Read the model definition and answer for the solid it produces. Units are mm, in the model's axes. Face numbers are marked on the shaded views. A direction names the side the tool comes from. Give positions to 0.01 mm unless a question says otherwise; leave off trailing zeros. Order: outer loops, then holes, each group sorted by start corner. A loop starts at its lowest first (then second) coordinate and runs counter-clockwise, first axis right, second up. Notation, with made-up numbers: (-10, 36) - (43, 36) arc R25 cw to (43, 51) - close; hole circle Ø2 at (5, -16). An arc over 180 degrees is marked (long way). Return JSON: item names as keys, results as strings.
```python
from build123d import *

# Parameters (mm, degrees)
SKETCH1_W                    = 410
SKETCH1_H                    = 200
BASE_FLANGE1_DEPTH           = 2
EDGE_FLANGE2_STRIP_W         = 13
EDGE_FLANGE2_STRIP_H         = 2
EDGE_FLANGE2_STRIP_CUT_DEPTH = 200
EDGE_FLANGE2_DEPTH           = 200
EDGE_FLANGE4_STRIP_W         = 13
EDGE_FLANGE4_STRIP_H         = 2
EDGE_FLANGE4_STRIP_CUT_DEPTH = 200
EDGE_FLANGE4_DEPTH           = 200
EDGE_FLANGE5_STRIP_W         = 13
EDGE_FLANGE5_STRIP_H         = 2
EDGE_FLANGE5_STRIP_CUT_DEPTH = 200
EDGE_FLANGE5_DEPTH           = 200
EDGE_FLANGE6_STRIP_W         = 13
EDGE_FLANGE6_STRIP_H         = 2
EDGE_FLANGE6_STRIP_CUT_DEPTH = 403
EDGE_FLANGE6_DEPTH           = 403
EDGE_FLANGE7_STRIP_W         = 13
EDGE_FLANGE7_STRIP_H         = 2
EDGE_FLANGE7_STRIP_CUT_DEPTH = 403
EDGE_FLANGE7_DEPTH           = 403
EDGE_FLANGE8_STRIP_W         = 13
EDGE_FLANGE8_STRIP_H         = 2
EDGE_FLANGE8_STRIP_CUT_DEPTH = 407.5
EDGE_FLANGE8_DEPTH           = 407.5
EDGE_FLANGE9_STRIP_W         = 13
EDGE_FLANGE9_STRIP_H         = 2
EDGE_FLANGE9_STRIP_CUT_DEPTH = 404.5
EDGE_FLANGE9_DEPTH           = 404.5
SKETCH29_R                   = 52.5
CUT_EXTRUDE1_DEPTH           = 10
SKETCH30_R                   = 3.25
CUT_EXTRUDE2_DEPTH           = 10


# Sheet-metal steps are written as plain solids
with BuildPart() as part:
    # Sketch1 → Base-Flange1 (new body)
    with BuildSketch(Plane.XY):
        with Locations((-14.494949495, 3.017676768)):
            Rectangle(SKETCH1_W, SKETCH1_H)
    extrude(amount=-BASE_FLANGE1_DEPTH)

    # Edge-Flange2 strip (across the edge) → Edge-Flange2 strip cut (cut)
    with BuildSketch(Plane(origin=(190.505050505, 103.017676768, -2), x_dir=(-1, 0, 0), z_dir=(0, -1, 0))):
        with Locations((-4, -1)):
            Rectangle(EDGE_FLANGE2_STRIP_W, EDGE_FLANGE2_STRIP_H)
    extrude(amount=EDGE_FLANGE2_STRIP_CUT_DEPTH, mode=Mode.SUBTRACT)

    # Edge-Flange2 section (across the edge) → Edge-Flange2 (add)
    with BuildSketch(Plane(origin=(190.505050505, 103.017676768, -2), x_dir=(-1, 0, 0), z_dir=(0, -1, 0))):
        with BuildLine():
            Line((-2, 2.5), (-2, 408))
            Line((-2, 408), (0, 408))
            Line((0, 408), (0, 2.5))
            ThreePointArc((0, 2.5), (0.732233047, 0.732233047), (2.5, 0))
            Line((2.5, 0), (2.5, -2))
            ThreePointArc((2.5, -2), (-0.681980515, -0.681980515), (-2, 2.5))
        make_face()
    extrude(amount=EDGE_FLANGE2_DEPTH)

    # Edge-Flange4 strip (across the edge) → Edge-Flange4 strip cut (cut)
    with BuildSketch(Plane(origin=(190.505050505, 103.017676768, -410), x_dir=(0, 0, 1), z_dir=(0, -1, 0))):
        with Locations((-4, -1)):
            Rectangle(EDGE_FLANGE4_STRIP_W, EDGE_FLANGE4_STRIP_H)
    extrude(amount=EDGE_FLANGE4_STRIP_CUT_DEPTH, mode=Mode.SUBTRACT)

    # Edge-Flange4 section (across the edge) → Edge-Flange4 (add)
    with BuildSketch(Plane(origin=(190.505050505, 103.017676768, -410), x_dir=(0, 0, 1), z_dir=(0, -1, 0))):
        with BuildLine():
            Line((-2, 2.5), (-2, 408))
            Line((-2, 408), (0, 408))
            Line((0, 408), (0, 2.5))
            ThreePointArc((0, 2.5), (0.732233047, 0.732233047), (2.5, 0))
            Line((2.5, 0), (2.5, -2))
            ThreePointArc((2.5, -2), (-0.681980515, -0.681980515), (-2, 2.5))
        make_face()
    extrude(amount=EDGE_FLANGE4_DEPTH)

    # Edge-Flange5 strip (across the edge) → Edge-Flange5 strip cut (cut)
    with BuildSketch(Plane(origin=(-217.494949495, 103.017676768, -410), x_dir=(1, 0, 0), z_dir=(0, -1, 0))):
        with Locations((-4, -1)):
            Rectangle(EDGE_FLANGE5_STRIP_W, EDGE_FLANGE5_STRIP_H)
    extrude(amount=EDGE_FLANGE5_STRIP_CUT_DEPTH, mode=Mode.SUBTRACT)

    # Edge-Flange5 section (across the edge) → Edge-Flange5 (add)
    with BuildSketch(Plane(origin=(-217.494949495, 103.017676768, -410), x_dir=(1, 0, 0), z_dir=(0, -1, 0))):
        with BuildLine():
            Line((-2, 2.5), (-2, 407))
            Line((-2, 407), (0, 407))
            Line((0, 407), (0, 2.5))
            ThreePointArc((0, 2.5), (0.732233047, 0.732233047), (2.5, 0))
            Line((2.5, 0), (2.5, -2))
            ThreePointArc((2.5, -2), (-0.681980515, -0.681980515), (-2, 2.5))
        make_face()
    extrude(amount=EDGE_FLANGE5_DEPTH)

    # Edge-Flange6 strip (across the edge) → Edge-Flange6 strip cut (cut)
    with BuildSketch(Plane(origin=(188.005050505, -96.982323232, -412), x_dir=(0, 1, 0), z_dir=(-1, 0, 0))):
        with Locations((-4, -1)):
            Rectangle(EDGE_FLANGE6_STRIP_W, EDGE_FLANGE6_STRIP_H)
    extrude(amount=EDGE_FLANGE6_STRIP_CUT_DEPTH, mode=Mode.SUBTRACT)

    # Edge-Flange6 section (across the edge) → Edge-Flange6 (add)
    with BuildSketch(Plane(origin=(188.005050505, -96.982323232, -412), x_dir=(0, 1, 0), z_dir=(-1, 0, 0))):
        with BuildLine():
            Line((-2, 2.5), (-2, 18))
            Line((-2, 18), (0, 18))
            Line((0, 18), (0, 2.5))
            ThreePointArc((0, 2.5), (0.732233047, 0.732233047), (2.5, 0))
            Line((2.5, 0), (2.5, -2))
            ThreePointArc((2.5, -2), (-0.681980515, -0.681980515), (-2, 2.5))
        make_face()
    extrude(amount=EDGE_FLANGE6_DEPTH)

    # Edge-Flange7 strip (across the edge) → Edge-Flange7 strip cut (cut)
    with BuildSketch(Plane(origin=(192.505050505, -96.982323232, -4.5), x_dir=(0, 1, 0), z_dir=(0, 0, -1))):
        with Locations((-4, -1)):
            Rectangle(EDGE_FLANGE7_STRIP_W, EDGE_FLANGE7_STRIP_H)
    extrude(amount=EDGE_FLANGE7_STRIP_CUT_DEPTH, mode=Mode.SUBTRACT)

    # Edge-Flange7 section (across the edge) → Edge-Flange7 (add)
    with BuildSketch(Plane(origin=(192.505050505, -96.982323232, -4.5), x_dir=(0, 1, 0), z_dir=(0, 0, -1))):
        with BuildLine():
            Line((-2, 2.5), (-2, 18))
            Line((-2, 18), (0, 18))
            Line((0, 18), (0, 2.5))
            ThreePointArc((0, 2.5), (0.732233047, 0.732233047), (2.5, 0))
            Line((2.5, 0), (2.5, -2))
            ThreePointArc((2.5, -2), (-0.681980515, -0.681980515), (-2, 2.5))
        make_face()
    extrude(amount=EDGE_FLANGE7_DEPTH)

    # Edge-Flange8 strip (across the edge) → Edge-Flange8 strip cut (cut)
    with BuildSketch(Plane(origin=(-219.494949495, -96.982323232, 0), x_dir=(0, 1, 0), z_dir=(1, 0, 0))):
        with Locations((-4, -1)):
            Rectangle(EDGE_FLANGE8_STRIP_W, EDGE_FLANGE8_STRIP_H)
    extrude(amount=EDGE_FLANGE8_STRIP_CUT_DEPTH, mode=Mode.SUBTRACT)

    # Edge-Flange8 section (across the edge) → Edge-Flange8 (add)
    with BuildSketch(Plane(origin=(-219.494949495, -96.982323232, 0), x_dir=(0, 1, 0), z_dir=(1, 0, 0))):
        with BuildLine():
            Line((-2, 2.5), (-2, 18))
            Line((-2, 18), (0, 18))
            Line((0, 18), (0, 2.5))
            ThreePointArc((0, 2.5), (0.732233047, 0.732233047), (2.5, 0))
            Line((2.5, 0), (2.5, -2))
            ThreePointArc((2.5, -2), (-0.681980515, -0.681980515), (-2, 2.5))
        make_face()
    extrude(amount=EDGE_FLANGE8_DEPTH)

    # Edge-Flange9 strip (across the edge) → Edge-Flange9 strip cut (cut)
    with BuildSketch(Plane(origin=(-219.494949495, -96.982323232, -407.5), x_dir=(0, 1, 0), z_dir=(0, 0, 1))):
        with Locations((-4, -1)):
            Rectangle(EDGE_FLANGE9_STRIP_W, EDGE_FLANGE9_STRIP_H)
    extrude(amount=EDGE_FLANGE9_STRIP_CUT_DEPTH, mode=Mode.SUBTRACT)

    # Edge-Flange9 section (across the edge) → Edge-Flange9 (add)
    with BuildSketch(Plane(origin=(-219.494949495, -96.982323232, -407.5), x_dir=(0, 1, 0), z_dir=(0, 0, 1))):
        with BuildLine():
            Line((-2, 2.5), (-2, 18))
            Line((-2, 18), (0, 18))
            Line((0, 18), (0, 2.5))
            ThreePointArc((0, 2.5), (0.732233047, 0.732233047), (2.5, 0))
            Line((2.5, 0), (2.5, -2))
            ThreePointArc((2.5, -2), (-0.681980515, -0.681980515), (-2, 2.5))
        make_face()
    extrude(amount=EDGE_FLANGE9_DEPTH)

    # Sketch29 → Cut-Extrude1 (cut)
    with BuildSketch(Plane.XY):
        with Locations((-15.744949495, 4.267676768)):
            Circle(SKETCH29_R)
    extrude(amount=-CUT_EXTRUDE1_DEPTH, mode=Mode.SUBTRACT)

    # Sketch30 → Cut-Extrude2 (cut)
    with BuildSketch(Plane(origin=(0, -96.982323232, 0), x_dir=(1, 0, 0), z_dir=(0, 1, 0))):
        with Locations(Location((-83.994949495, -10.25, 0), (0, 0, 270))):
            Circle(SKETCH30_R)
        with Locations(Location((52.505050505, -10.25, 0), (0, 0, 270))):
            Circle(SKETCH30_R)
        with Locations(Location((202.755050505, 140, 0), (0, 0, 270))):
            Circle(SKETCH30_R)
        with Locations(Location((202.755050505, 276.5, 0), (0, 0, 270))):
            Circle(SKETCH30_R)
        with Locations(Location((52.505050505, 422.25, 0), (0, 0, 270))):
            Circle(SKETCH30_R)
        with Locations(Location((-83.994949495, 422.25, 0), (0, 0, 270))):
            Circle(SKETCH30_R)
        with Locations(Location((-229.744949495, 272, 0), (0, 0, 270))):
            Circle(SKETCH30_R)
        with Locations(Location((-229.744949495, 135.5, 0), (0, 0, 270))):
            Circle(SKETCH30_R)
    extrude(amount=-CUT_EXTRUDE2_DEPTH, mode=Mode.SUBTRACT)


solid = part.part
```
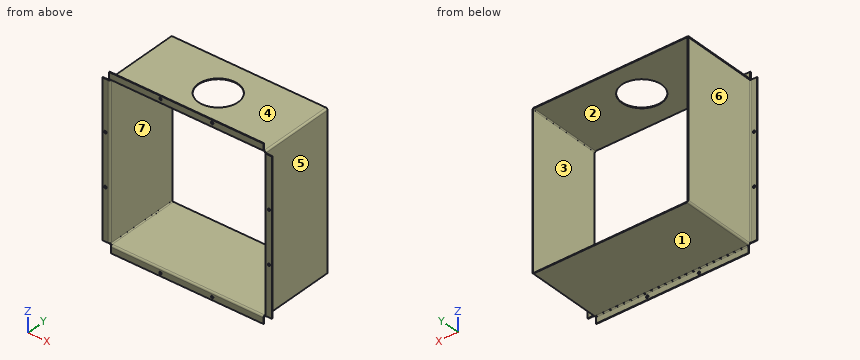
Q1. Given pin 1 (3.5 mm diameter, centred on x = 191.5, z = -409, fed in from -Y); pin 2 (0.6 mm diameter, centred on y = -96, z = -1.5, fed in from -X); pin 3 (10 mm diameter, centred on x = -224, y = -20.5, fed in from +Z), each flat-ended and moving along its own axis, determine where each tip first touches the part or whether it passes through.
Values:
{"pin 1": "stops at y = -98.15", "pin 2": "stops at x = -219.49", "pin 3": "stops at z = 0"}
Q2. Consider L1, parallel to Z at x = 34, y = 24; L2, parallel to X at y = 66, z = -131.5; L3, parallel to X at y = -98.6, z = -272. Determine where each line is inside the solid, lowest interval first.
Values:
{"L1": "z = -412 to -410, -2 to 0", "L2": "x = -219.49 to -217.49, 190.51 to 192.51", "L3": "x = -237.49 to -232.99, -226.49 to -220.18, 193.19 to 210.51"}
Q3. A cutting plane is placed at C-C (y = -2.5). Write down the section's boundary in (x, z), and give its area (3 significant figures).
Values:
{"outline": "(-219.49, -407.5) arc R4.5 ccw to (-214.99, -412) - (188.01, -412) arc R4.5 ccw to (192.51, -407.5) - (192.51, -4.5) arc R4.5 ccw to (188.01, 0) - (36.32, 0) - (36.32, -2) - (188.01, -2) arc R2.5 cw to (190.51, -4.5) - (190.51, -407.5) arc R2.5 cw to (188.01, -410) - (-214.99, -410) arc R2.5 cw to (-217.49, -407.5) - (-217.49, -3) - (-219.49, -3) - close; (-219.49, -2) - (-67.81, -2) - (-67.81, 0) - (-219.49, 0) - close", "area": "3,060 mm²"}
Q4. Determine the mould class of the marked faces 1, 2, 3 and 4 for opening direction Z: released by +Z, released by -Z, zero draft, split by the parting line, or undercut.
Values:
{"face 1": "released by -Z", "face 2": "undercut", "face 3": "undercut", "face 4": "released by +Z"}
Q5. A cutting plane is placed at B-B (z = -220.5). Write down the section's boundary in (x, y), and give its area (3 significant figures).
Values:
{"outline": "(-237.49, -98.98) - (-221.99, -98.98) arc R4.5 ccw to (-217.49, -94.48) - (-217.49, 103.02) - (-219.49, 103.02) - (-219.49, -94.48) arc R2.5 cw to (-221.99, -96.98) - (-237.49, -96.98) - close; (190.51, -94.48) arc R4.5 ccw to (195.01, -98.98) - (210.51, -98.98) - (210.51, -96.98) - (195.01, -96.98) arc R2.5 cw to (192.51, -94.48) - (192.51, 103.02) - (190.51, 103.02) - close", "area": "874 mm²"}
Q6. For the marked faces 5, 6 and 7, determine the directions among +Z, -Z, +X, -X, +Y, -Y from which every point of the face is accessible in a straight line to the end or side of a thin tool.
Values:
{"face 5": "+Z, -Z, +X, +Y", "face 6": "+Z, -Z, -X, +Y", "face 7": "+Y, -Y"}
Q7. A cutting plane is placed at A-A (x = -115). Write down the section's boundary in (y, z), and give its area (3 significant figures).
Values:
{"outline": "(-98.98, -430) - (-96.98, -430) - (-96.98, -414.5) arc R2.5 cw to (-94.48, -412) - (103.02, -412) - (103.02, -410) - (-94.48, -410) arc R4.5 ccw to (-98.98, -414.5) - close; (-98.98, 2.5) arc R4.5 ccw to (-94.48, -2) - (103.02, -2) - (103.02, 0) - (-94.48, 0) arc R2.5 cw to (-96.98, 2.5) - (-96.98, 18) - (-98.98, 18) - close", "area": "874 mm²"}
